from build123d import *

# Parameters (mm, degrees)
SKETCH_1_W               = 57.1
SKETCH_1_H               = 80.7
EXTRUDE_1_DEPTH          = 7.1
SKETCH_3_W               = 57.1
SKETCH_3_H               = 8
CUT_EXTRUDE_2_DEPTH      = 4.8
CUT_EXTRUDE_3_DEPTH      = 100.112612719
SKETCH_5_W               = 1.6
SKETCH_5_H               = 4
CUT_EXTRUDE_4_DEPTH      = 100.112612719
SKETCH_6_W               = 1.6
SKETCH_6_H               = 4
EXTRUDE_2_DEPTH          = 7.1
SKETCH_7_W               = 2.6
SKETCH_7_H               = 47.6
SKETCH_7_H_2             = 38.5
EXTRUDE_3_DEPTH          = 8.2
SKETCH_8_W               = 12
SKETCH_8_H               = 16.3
EXTRUDE_4_DEPTH          = 10.5
SKETCH_9_W               = 4.45
SKETCH_9_H               = 3
EXTRUDE_5_DEPTH          = 10.5
SKETCH_10_W              = 8.9
SKETCH_10_H              = 10.4
EXTRUDE_6_DEPTH          = 10.5
FILLET_1_R               = 4.5
CUT_EXTRUDE_7_DEPTH      = 101.034943895
CUT_EXTRUDE_7_DEPTH_BACK = 101.034943895
SKETCH_11_R              = 1.5


with BuildPart() as part:
    # 草图1 → 凸台-拉伸1 (new body)
    with BuildSketch(Plane(origin=(0, 0, 0), x_dir=(1, 0, 0), z_dir=(0, 1, 0))):
        with Locations((28.55, 40.35)):
            Rectangle(SKETCH_1_W, SKETCH_1_H)
    extrude(amount=EXTRUDE_1_DEPTH)

    # 草图3 → 切除-拉伸2 (cut)
    with BuildSketch(Plane(origin=(0, 7.1, 0), x_dir=(1, 0, 0), z_dir=(0, 1, 0))):
        with Locations((28.55, 76.7)):
            Rectangle(SKETCH_3_W, SKETCH_3_H)
    extrude(amount=-CUT_EXTRUDE_2_DEPTH, mode=Mode.SUBTRACT)

    # 草图4 → 切除-拉伸3 (cut, through all)
    with BuildSketch(Plane(origin=(0, 7.1, 0), x_dir=(1, 0, 0), z_dir=(0, 1, 0))):
        with BuildLine():
            Line((57.1, 0), (57.1, 2.5))
            Line((57.1, 2.5), (42.31941151, 2.5))
            ThreePointArc((42.31941151, 2.5), (42.118493782, 2.457855945), (41.951446004, 2.338528265))
            Line((41.951446004, 2.338528265), (39.8, 0))
            Line((39.8, 0), (57.1, 0))
        make_face()
        with BuildLine():
            Line((0, 2.5), (4.292893219, 2.5))
            ThreePointArc((4.292893219, 2.5), (4.484234935, 2.461939766), (4.646446609, 2.353553391))
            Line((4.646446609, 2.353553391), (7, 0))
            Line((7, 0), (0, 0))
            Line((0, 0), (0, 2.5))
        make_face()
    extrude(amount=-CUT_EXTRUDE_3_DEPTH, mode=Mode.SUBTRACT)

    # 草图5 → 切除-拉伸4 (cut, through all)
    with BuildSketch(Plane(origin=(0, 7.1, 0), x_dir=(1, 0, 0), z_dir=(0, 1, 0))):
        with Locations((56.3, 40.3)):
            Rectangle(SKETCH_5_W, SKETCH_5_H)
    extrude(amount=-CUT_EXTRUDE_4_DEPTH, mode=Mode.SUBTRACT)

    # 草图6 → 凸台-拉伸2 (add)
    with BuildSketch(Plane(origin=(0, 7.1, 0), x_dir=(1, 0, 0), z_dir=(0, 1, 0))):
        with Locations((-0.8, 40.3)):
            Rectangle(SKETCH_6_W, SKETCH_6_H)
    extrude(amount=-EXTRUDE_2_DEPTH)

    # 草图7 → 凸台-拉伸3 (add)
    with BuildSketch(Plane(origin=(0, 7.1, 0), x_dir=(1, 0, 0), z_dir=(0, 1, 0))):
        with Locations((52.4, 29.3)):
            Rectangle(SKETCH_7_W, SKETCH_7_H)
        with Locations((4.7, 24.75)):
            Rectangle(SKETCH_7_W, SKETCH_7_H_2)
    extrude(amount=EXTRUDE_3_DEPTH)

    # 草图8 → 凸台-拉伸4 (add)
    with BuildSketch(Plane(origin=(0, 7.1, 0), x_dir=(1, 0, 0), z_dir=(0, 1, 0))):
        with Locations((39.9, 68.85)):
            Rectangle(SKETCH_8_W, SKETCH_8_H)
    extrude(amount=EXTRUDE_4_DEPTH)

    # 草图9 → 凸台-拉伸5 (add)
    with BuildSketch(Plane(origin=(0, 7.1, 0), x_dir=(1, 0, 0), z_dir=(0, 1, 0))):
        with Locations((13.875, 71.2)):
            Rectangle(SKETCH_9_W, SKETCH_9_H)
        with Locations((9.425, 71.2)):
            Rectangle(SKETCH_9_W, SKETCH_9_H)
    extrude(amount=EXTRUDE_5_DEPTH)

    # 草图10 → 凸台-拉伸6 (add)
    with BuildSketch(Plane(origin=(0, 7.1, 0), x_dir=(1, 0, 0), z_dir=(0, 1, 0))):
        with Locations((11.65, 64.5)):
            Rectangle(SKETCH_10_W, SKETCH_10_H)
    extrude(amount=EXTRUDE_6_DEPTH)

    # 圆角1
    # the kernel refuses this fillet: 4.5 mm, written as the material it takes off along each edge
    with BuildSketch(Plane(origin=(7.2, 17.6, -48.05), x_dir=(0, -1, 0), z_dir=(0, 0, -1))) as fillet_1_piece_1:
        with BuildLine():
            CenterArc((FILLET_1_R, -FILLET_1_R), FILLET_1_R, 90, 90)
            Line((0, -FILLET_1_R), (0, 0))
            Line((0, 0), (FILLET_1_R, 0))
        make_face()
    extrude(amount=35.9, mode=Mode.SUBTRACT)
    with BuildSketch(Plane(origin=(16.1, 17.6, -83.95), x_dir=(-1, 0, 0), z_dir=(0, 0, 1))) as fillet_1_piece_2:
        with BuildLine():
            CenterArc((FILLET_1_R, FILLET_1_R), FILLET_1_R, 180, 90)
            Line((0, FILLET_1_R), (0, 0))
            Line((0, 0), (FILLET_1_R, 0))
        make_face()
    extrude(amount=35.9, mode=Mode.SUBTRACT)

    # 草图11 → 切除-拉伸7 (cut, two sides: drawn at the far end of the back side and taken through both)
    with BuildSketch(Plane(origin=(0, 2.3, 0), x_dir=(1, 0, 0), z_dir=(0, 1, 0)).offset(-CUT_EXTRUDE_7_DEPTH_BACK)):
        with Locations(Location((52.9, 77.1, 0), (0, 0, 270))):
            Circle(SKETCH_11_R)
        with Locations(Location((4.2, 77.1, 0), (0, 0, 270))):
            Circle(SKETCH_11_R)
        with Locations(Location((37.1, 4.6, 0), (0, 0, 270))):
            Circle(SKETCH_11_R)
        with Locations(Location((9, 4.6, 0), (0, 0, 270))):
            Circle(SKETCH_11_R)
    extrude(amount=CUT_EXTRUDE_7_DEPTH + CUT_EXTRUDE_7_DEPTH_BACK, mode=Mode.SUBTRACT)


solid = part.part
Can you work these out from the model? Positions are in its coordinate system, mm. A direction names the side the tool comes from. Coordinates: 2 decimals unless noted, no trailing zeros. Write each loop counter-clockwise with the first axis right and the second up, starting at its lowest first coordinate (ties: lowest second). Pieces come first, ordered by that corner, then holes. Notation, with made-up numbers: (39, 33.5) -> (87, 33.5) arc R29 cw to (87, 59.5) -> close; hole circle Ø9 at (-25, -13.75). An arc over 180 degrees is marked (long way). Answer as CSV lines item,"result".
1) If we section it at B-B on z = -4.6: Please give me the cut outline in (x, y).
Check result:
outline,"(0, 0) -> (7.5, 0) -> (7.5, 7.1) -> (0, 7.1) -> close; (10.5, 0) -> (35.6, 0) -> (35.6, 7.1) -> (10.5, 7.1) -> close; (38.6, 0) -> (57.1, 0) -> (57.1, 7.1) -> (38.6, 7.1) -> close"
2) Will these pins go through, and if not, where does the flat tip stop? P1, Ø8, axis at y = 4.5, z = -12, coming from the -X side; P2, Ø1.3, axis at x = 2, y = 3.5, coming from the +Z side; P3, Ø8, axis at x = 42, y = 11, coming from the -Z side; P4, Ø2.5, axis at x = 37.1, z = -4.6, coming from the -Y side.
Check result:
P1,"x = 0"
P2,"z = -2.5"
P3,"z = -77"
P4,"through"
3) If we section it at C-C on z = -47: Please give me the cut outline in (x, y).
Check result:
outline,"(0, 0) -> (57.1, 0) -> (57.1, 7.1) -> (53.7, 7.1) -> (53.7, 15.3) -> (51.1, 15.3) -> (51.1, 7.1) -> (0, 7.1) -> close"
4) If we section it at A-A on x = 37.1: Please give me the cut outline in (y, z).
Check result:
outline,"(0, -80.7) -> (2.3, -80.7) -> (2.3, -72.7) -> (7.1, -72.7) -> (7.1, -77) -> (17.6, -77) -> (17.6, -60.7) -> (7.1, -60.7) -> (7.1, -6.1) -> (0, -6.1) -> close; (0, -3.1) -> (7.1, -3.1) -> (7.1, 0) -> (0, 0) -> close"
5) If we section it at D-D on x = 49: Please give me the cut outline in (y, z), then the cut area to 3 significant figures.
Check result:
outline,"(0, -80.7) -> (2.3, -80.7) -> (2.3, -72.7) -> (7.1, -72.7) -> (7.1, -2.5) -> (0, -2.5) -> close"
area,"517 mm²"
6) On a 3-axis mill with a long thin cutter (end or side, diameter ignored), from which of +Z, -Z, +X, -X, +Y, -Y can I reach the whole of each face in a straight line? I mean faces 4 (the flat face through (12, 12, -59.3)), 5 (the flat face through (0, 4, -57)), 6 (the flat face through (53.7, 11, -29)), 7 (the flat face through (55.5, 4, -40)). Say none if no direction works.
Check result:
face 4,"+Z, +X, -X, +Y"
face 5,"-Z, -X, +Y, -Y"
face 6,"+Z, -Z, +X, +Y"
face 7,"+X, +Y, -Y"
7) If I drill on line 1 (X direction, y = 0.7, z = -77.1); line 2 (X direction, y = 5.5, z = -4.6); line 3 (Z direction, x = 4.2, y = 0.6), over which ranges is the centre line in solid material (lowest first)? Write a range as from..to.
Check result:
line 1,"0..2.7, 5.7..51.4, 54.4..57.1"
line 2,"0..7.5, 10.5..35.6, 38.6..57.1"
line 3,"-80.7..-78.6, -75.6..-2.5"
8) If we mould it in two halves opening along Z, with no side actions, what happens to faces 1 (the cylindrical face through (52.97, 1.13, -78.6)), 2 (the flat face through (33.9, 12, -69)), 3 (the flat face through (5, 11, -44))? For each: +Z half, -Z half, draft (parallel to the pull), parting line (faces both ways), or undercut.
Check result:
face 1,"undercut"
face 2,"draft"
face 3,"-Z half"
